Work out the finished part from the listing and answer in its coordinate system (mm). Give positions to 0.01 mm unless a question says otherwise; leave off trailing zeros. Loops run counter-clockwise (first coordinate to the right, second up) from the corner with the lowest first, then second, coordinate; pieces in that order, holes last. Notation, with made-up numbers: M 4,0.5 L 23,0.5 A9 cw 23,17.5 Z; hole C -24.5,-13 d8. An arc over 180 degrees is marked long. Write item = value, one per line. Start each with the question number.
1. Section A-A on x = -0.5 is taken. Determine the outline of the cut face in (y, z).
2. Section B-B on y = 149 is taken. Determine the outline of the cut face in (x, z).
3. Consider L1, parallel to Z at x = -0.9, y = 168; L2, parallel to X at y = 120, z = -2.4; L3, parallel to Z at x = -0.35, y = 100. Determine where each line is inside the solid, lowest interval first. Write a range as [from, to].
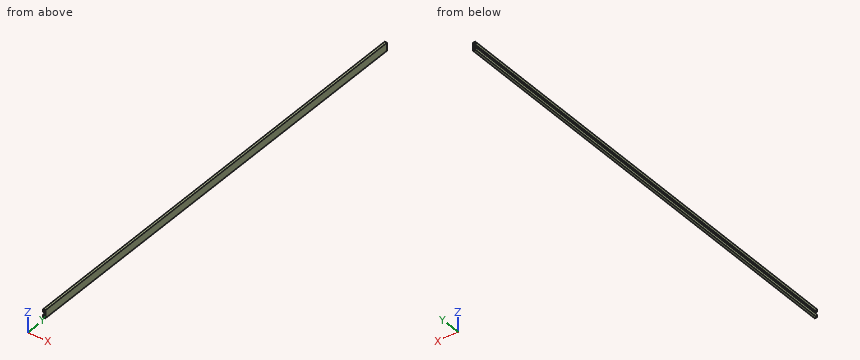
Autodesk Inventor part; units mm, degrees
ref_plane "YZ Plane" through (0, 0, 0) normal (1, 0, 0) x (0, 1, 0)
ref_plane "XZ Plane" through (0, 0, 0) normal (0, 1, 0) x (-1, 0, 0)
ref_plane "XY Plane" through (0, 0, 0) normal (0, 0, 1) x (1, 0, 0)
sketch "Skizze2" plane through (0, 0, 0) normal (0, 1, 0) x (-1, 0, 0)
  line L0 (0, 0) -> (1, 0) construction
  line L1 (1, 0) -> (1, -3.4) construction
  line L2 (1, -3.4) -> (0, -3.4) construction
  line L3 (0, -3.4) -> (0, 0) construction
  line L4 (0.7, -3.1) -> (0.7, -0.3) construction
  line L5 (0.7, -0.3) -> (0.3, -0.3) construction
  line L6 (0.3, -0.3) -> (0.3, -3.1) construction
  line L7 (0.3, -3.1) -> (0.7, -3.1) construction
  line L8 (1, -1.7) -> (0, -1.7) construction
  line L9 (1, -1.2) -> (0.7, -1.2)
  line L10 (1, -2.2) -> (0.7, -2.2)
  line L11 (1, -1.2) -> (1, 0)
  line L12 (0, 0) -> (0, -3.4)
  line L13 (1, -3.4) -> (1, -2.2)
  line L14 (0.7, -2.2) -> (0.7, -3.1)
  line L15 (0.3, -3.1) -> (0.3, -0.3)
  line L16 (0.7, -0.3) -> (0.7, -1.2)
  line L17 (0.7, -0.3) -> (0.3, -0.3)
  line L18 (1, 0) -> (0, 0)
  line L19 (0.3, -3.1) -> (0.7, -3.1)
  line L20 (1, -3.4) -> (0, -3.4)
  dimension "d0" = 1
  dimension "d1" = 3.4
  dimension "d2" = 0.3
  dimension "d3" = 0.5
  dimension "d4" = 0.5
extrude "Extrusion1" add sketch "Skizze2" along normal blind 197.5
equation "\"Biegeradius\" = Stärke"
equation "\"BreiteBiegungsfreistellung\" = Stärke"
equation "\"TiefeBiegungsfreistellung\" = 0.5 * Stärke"
equation "\"GrößeEckenfreistellung\" = 4 * Stärke"
equation "\"MinimalRest\" = 2 * Stärke"
equation "\"Übergangsradius\" = Biegeradius"
equation "\"JacobiRadiusGröße\" = Biegeradius"
equation "\"Abstandsgröße\" = Stärke"
properties part number "Boden_airline_eckig"
Verdict:
q1.outline = M 0,-3.4 L 197.5,-3.4 L 197.5,-3.1 L 0,-3.1 Z; M 0,-0.3 L 197.5,-0.3 L 197.5,0 L 0,0 Z
q2.outline = M -1,-3.4 L 0,-3.4 L 0,0 L -1,0 L -1,-1.2 L -0.7,-1.2 L -0.7,-0.3 L -0.3,-0.3 L -0.3,-3.1 L -0.7,-3.1 L -0.7,-2.2 L -1,-2.2 Z
q3.L1 = [-3.4, -2.2], [-1.2, 0]
q3.L2 = [-1, -0.7], [-0.3, 0]
q3.L3 = [-3.4, -3.1], [-0.3, 0]
